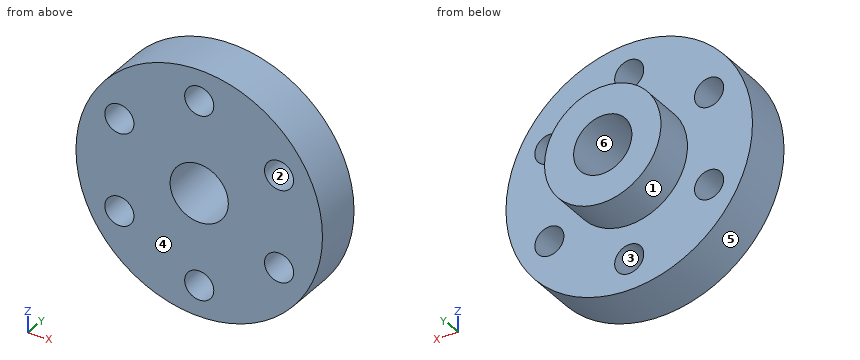
Autodesk Inventor part; units mm, degrees
ref_plane "YZ Plane" through (0, 0, 0) normal (1, 0, 0) x (0, 1, 0)
ref_plane "XZ Plane" through (0, 0, 0) normal (0, 1, 0) x (-1, 0, 0)
ref_plane "XY Plane" through (0, 0, 0) normal (0, 0, 1) x (1, 0, 0)
sketch "Esquisse1" plane through (0, 0, 0) normal (0, 1, 0) x (-1, 0, 0)
  circle A0 centre (0, 0) radius 12.7
  dimension "d0" = 25.4
extrude "Extrusion1" add sketch "Esquisse1" along normal blind 5
sketch "Esquisse2" plane through (0, 5, 0) normal (0, 1, 0) x (1, 0, 0)
  circle A0 centre (0, 0) radius 12.7
  circle A1 centre (0, 0) radius 6
  dimension "d3" = 12
extrude "Extrusion2" add sketch "Esquisse2" along normal blind 4.2 contours A1
sketch "Esquisse3" plane through (0, 9.2, 0) normal (0, 1, 0) x (1, 0, 0)
  circle A0 centre (0, 0) radius 6
  circle A1 centre (0, 0) radius 3
  dimension "d6" = 6
extrude "Extrusion3" cut sketch "Esquisse3" against normal through all contours A1
sketch "Esquisse4" plane through (0, 0, 0) normal (0, -1, 0) x (1, 0, 0)
  circle A0 centre (0, 0) radius 3
  circle A1 centre (0, 9.5) radius 1.5
  circle A2 centre (-8.2272, 4.75) radius 1.5
  circle A3 centre (-8.2272, -4.75) radius 1.5
  circle A4 centre (0, -9.5) radius 1.5
  circle A5 centre (8.2272, -4.75) radius 1.5
  circle A6 centre (8.2272, 4.75) radius 1.5
  dimension "d9" = 3
  dimension "d10" = 9.5
  dimension "d11" = 0
  dimension "d14" = 360
extrude "Extrusion4" cut sketch "Esquisse4" against normal through all contours A1 | A2 | A3 | A4 | A5 | A6
properties part number "hub_6mm_M3"
Input: part model. Units: mm. Frame: model coordinates. Face numbers are marked on the shaded views. A direction names the side the tool comes from. Coordinates: 2 decimals unless noted, no trailing zeros. Loops run counter-clockwise (first coordinate to the right, second up) from the corner with the lowest first, then second, coordinate; pieces in that order, holes last.
(1) Set-up query: the marked faces 1 and 2. Return all of +Z, -Z, +X, -X, +Y, -Y with unobstructed straight access to the full face (end or side cutting, diameter ignored); none if empty.
(2) Section B-B on y = 1. Return the cut outline in (x, z).
(3) Section C-C on z = 4.75. Return the cut outline in (x, y), then the cut area to 3 significant figures.
(4) Material intervals for probe 1 along Z at (x, y) = (0, 3.65); probe 2 along Y at (x, z) = (-5, -8.75); probe 3 along X at (y, z) = (1, -1.25), sorted ascending.
(5) Pull-direction query (X, two-part tool) for the marked faces 3, 4, 5 and 6; classes: released by +X, released by -X, zero draft, split by the parting line, or undercut.
(6) Section A-A on x = 0. Return the cut outline in (y, z), then the cut area to 3 significant figures.
(7) First-contact query: pin 1 Ø1 at (x, z) = (-5.5, -7.5) entering from +Y; pin 2 Ø5 at (y, z) = (6, -8) entering from -X; pin 3 Ø4 at (y, z) = (6, -6) entering from +X. Flat tips, straight axial feed; report the tip coordinate or a pass-through.
(8) Section D-D on z = 0. Return the cut outline in (x, y), then the cut area to 3 significant figures.
Data:
1. face 1: +Y
1. face 2: +Y, -Y
2. outline: circle Ø25.4 at (0, 0); hole circle Ø3 at (-8.23, -4.75); hole circle Ø3 at (-8.23, 4.75); hole circle Ø6 at (0, 0); hole circle Ø3 at (0, -9.5); hole circle Ø3 at (0, 9.5); hole circle Ø3 at (8.23, -4.75); hole circle Ø3 at (8.23, 4.75)
3. outline: (-11.78, 0) - (-9.73, 0) - (-9.73, 5) - (-11.78, 5) - close; (-6.73, 0) - (6.73, 0) - (6.73, 5) - (3.67, 5) - (3.67, 9.2) - (-3.67, 9.2) - (-3.67, 5) - (-6.73, 5) - close; (9.73, 0) - (11.78, 0) - (11.78, 5) - (9.73, 5) - close
3. area: 119 mm2
4. probe 1: z = -12.7 to -11, -8 to -3, 3 to 8, 11 to 12.7
4. probe 2: y = 0 to 5
4. probe 3: x = -12.64 to -2.73, 2.73 to 12.64
5. face 3: undercut
5. face 4: zero draft
5. face 5: split by the parting line
5. face 6: undercut
6. outline: (0, -12.7) - (5, -12.7) - (5, -11) - (0, -11) - close; (0, -8) - (5, -8) - (5, -6) - (9.2, -6) - (9.2, -3) - (0, -3) - close; (0, 3) - (9.2, 3) - (9.2, 6) - (5, 6) - (5, 8) - (0, 8) - close; (0, 11) - (5, 11) - (5, 12.7) - (0, 12.7) - close
6. area: 92.2 mm2
7. pin 1: stops at y = 5
7. pin 2: stops at x = -11.34
7. pin 3: stops at x = 11.96
8. outline: (-12.7, 0) - (-3, 0) - (-3, 9.2) - (-6, 9.2) - (-6, 5) - (-12.7, 5) - close; (3, 0) - (12.7, 0) - (12.7, 5) - (6, 5) - (6, 9.2) - (3, 9.2) - close
8. area: 122 mm2
